The listing builds one solid part. Answer for the finished solid, in the listing's coordinates (mm). Face numbers are marked on the shaded views. A direction names the side the tool comes from. Give positions to 0.01 mm unless a question says otherwise; leave off trailing zeros. Order: outer loops, then holes, each group sorted by start corner. A loop starts at its lowest first (then second) coordinate and runs counter-clockwise, first axis right, second up. Notation, with made-up numbers: (69.5, 33) - (75.5, 33) arc R10 cw to (75.5, 39) - close; hole circle Ø9 at (48, 37). An arc over 180 degrees is marked (long way). Write each question's results on one line, items separated by ' | '. Start each with the question number.
1. Find the intervals of material crossed by L1, parallel to Y at x = 15, z = 3.5; L2, parallel to Y at x = 18.75, z = -3.25; L3, parallel to Y at x = 15, z = 2.5, in increasing order.
2. Section B-B (x = 15) is taken. Give the vertices of the cut face in (y, z).
3. Section A-A (y = 26) is taken. Give the vertices of the cut face in (x, z).
4. Flat-ended cylindrical pins translate along their axes: pin 1 (1.8 mm diameter, centred on x = 16, y = 21, fed in from -Z); pin 2 (3 mm diameter, centred on x = 15, y = 24, fed in from +Z); pin 3 (6.5 mm diameter, centred on y = -3.5, z = 1, fed in from -X); pin 4 (6 mm diameter, centred on y = 24, z = 4.5, fed in from +X). Find the tip coordinate at first contact, or state that the pin passes through.
5. Section D-D (x = 11.5) is taken. Give the vertices of the cut face in (y, z), and give its area (3 significant figures).
6. Determine the mould class of the marked faces 1, 2, 3 and 4 for opening direction Y: released by +Y, released by -Y, zero draft, split by the parting line, or undercut.
7. Which of the six approach directions +Z, -Z, +X, -X, +Y, -Y give full straight-line access (tool end or side, diameter ignored) to the marked faces 5, 6, 7, 8 and 9?
8. Section C-C (z = -0.5) is taken. Give the vertices of the cut face in (x, y).
Autodesk Inventor part; units mm, degrees
ref_plane "YZ Plane" through (0, 0, 0) normal (1, 0, 0) x (0, 1, 0)
ref_plane "XZ Plane" through (0, 0, 0) normal (0, 1, 0) x (-1, 0, 0)
ref_plane "XY Plane" through (0, 0, 0) normal (0, 0, 1) x (1, 0, 0)
sketch "스케치1" plane through (0, 0, 0) normal (0, 0, 1) x (1, 0, 0)
  line L0 (0, 0) -> (30, 0)
  line L1 (30, 0) -> (30, 20)
  line L2 (30, 20) -> (0, 20)
  line L3 (0, 20) -> (0, 0)
  line L4 (0, 20) -> (30, 20)
  line L5 (30, 20) -> (30, 17)
  line L6 (0, 17) -> (0, 20)
  line L7 (12, 20) -> (18, 20)
  line L8 (18, 20) -> (18, 16)
  line L9 (18, 16) -> (12, 16)
  line L10 (12, 16) -> (12, 20)
  point P0 (15, 20)
  point P1 (15, 20)
  dimension "d0" = 20
  dimension "d1" = 30
  dimension "d2" = 3
  dimension "d3" = 6
  dimension "d4" = 4
extrude "돌출1" add sketch "스케치1" along normal blind 10 contours L2 L8 L9 L10
sketch "스케치2" plane through (0, 0, 10) normal (0, 0, 1) x (1, 0, 0)
  line L0 (18, 20) -> (12, 20)
  line L1 (12, 20) -> (18, 20)
  line L2 (18, 20) -> (18, -3)
  line L3 (18, -3) -> (12, -3)
  line L4 (12, -3) -> (12, 20)
  point P0 (0, 0)
  dimension "d23" = 23
extrude "돌출2" add sketch "스케치2" along normal blind 4
sketch "스케치3" plane through (0, 0, 10) normal (0, 0, -1) x (-1, 0, 0)
  line L0 (-18, -3) -> (-18, 16)
  line L1 (-12, 16) -> (-12, -3)
  line L2 (-18, -3) -> (-12, -3)
  line L3 (-12, -3) -> (-12, 1)
  line L4 (-12, 1) -> (-18, 1)
  line L5 (-18, 1) -> (-18, -3)
  point P0 (0, 0)
  dimension "d9" = 4
extrude "돌출3" add sketch "스케치3" along normal blind 15
sketch "스케치6" plane through (0, 0, 0) normal (0, 0, -1) x (-1, 0, 0)
  line L0 (-18, 16) -> (-18, 20)
  line L1 (-12, 16) -> (-18, 16)
  line L2 (-12, 20) -> (-12, 16)
  line L3 (-18, 20) -> (-12, 20)
  line L4 (-18, 16) -> (-18, 20)
  line L5 (-18, 16) -> (-12, 16)
  line L6 (-12, 16) -> (-12, 36)
  line L7 (-12, 36) -> (-18, 36)
  line L8 (-18, 36) -> (-18, 16)
  point P0 (0, 0)
  dimension "d20" = 20
extrude "돌출6" add sketch "스케치6" against normal blind 4 contours L8 L7 L6 L3
sketch "스케치7" plane through (12, 1, 10) normal (0, 1, 0) x (1, 0, 0)
  line L0 (6, 0) -> (0, 0)
  line L1 (6, 0) -> (6, 15)
  line L2 (0, 15) -> (6, 15)
  line L3 (0, 0) -> (0, 15)
  line L4 (-4.5, 15) -> (10.5, 15)
  line L5 (10.5, 15) -> (10.5, 10)
  line L6 (10.5, 10) -> (-4.5, 10)
  line L7 (-4.5, 10) -> (-4.5, 15)
  point P0 (-12, 10)
  point P1 (3, 15)
  point P2 (3, 15)
  point P3 (6, 15)
  point P4 (6, 10)
  point P5 (0, 10)
  dimension "d27" = 15
extrude "돌출7" add sketch "스케치7" against normal blind 4 contours L1 L4 L5 L6 | L6 L7 L4 L3
sketch "스케치8" plane through (0, 0, -5) normal (0, 0, -1) x (-1, 0, 0)
  line L0 (-22.5, 1) -> (-7.5, 1)
  line L1 (-22.5, 1) -> (-22.5, -3)
  line L2 (-7.5, -3) -> (-22.5, -3)
  line L3 (-7.5, 1) -> (-7.5, -3)
  line L4 (-22.5, 1) -> (-7.5, 1)
  line L5 (-7.5, 1) -> (-7.5, -6)
  line L6 (-7.5, -6) -> (-22.5, -6)
  line L7 (-22.5, -6) -> (-22.5, 1)
  point P0 (0, 0)
  dimension "d28" = 7
extrude "돌출8" add sketch "스케치8" against normal blind 10
sketch "스케치9" plane through (0, 0, -5) normal (0, 0, -1) x (-1, 0, 0)
  line L0 (-20.1, 0.5) -> (-9.9, 0.5)
  line L1 (-9.9, 0.5) -> (-9.9, -4.5)
  line L2 (-9.9, -4.5) -> (-20.1, -4.5)
  line L3 (-20.1, -4.5) -> (-20.1, 0.5)
  line L4 (-22.5, 1) -> (-7.5, 1)
  line L5 (-22.5, 1) -> (-22.5, -6)
  point P0 (0, 0)
  point P1 (-15, 1)
  point P2 (-15, 0.5)
  dimension "d31" = 10.2
  dimension "d32" = 5
  dimension "d33" = 0.5
extrude "돌출9" cut sketch "스케치9" against normal blind 8
sketch "스케치10" plane through (0, 0, -5) normal (0, 0, -1) x (-1, 0, 0)
  line L0 (-9.9, 0.5) -> (-9.9, -4.5)
  line L1 (-9.9, -4.5) -> (-20.1, -4.5)
  line L2 (-20.1, -4.5) -> (-20.1, 0.5)
  line L3 (-20.1, 0.5) -> (-9.9, 0.5)
  line L4 (-22.5, 1) -> (-7.5, 1)
  line L5 (-22.5, 1) -> (-22.5, -6)
  line L6 (-22.5, -6) -> (-7.5, -6)
  line L7 (-7.5, 1) -> (-7.5, -6)
  point P0 (0, 0)
extrude "돌출10" add sketch "스케치10" along normal blind 2
sketch "스케치11" plane through (12, 1, 10) normal (0, 1, 0) x (1, 0, 0)
  line L0 (0, 0) -> (0, 5)
  line L1 (6, 0) -> (0, 0)
  line L2 (6, 0) -> (6, 5)
  line L3 (10.5, 5) -> (6, 5)
  line L4 (10.5, 5) -> (10.5, 17)
  line L5 (-4.5, 17) -> (10.5, 17)
  line L6 (-4.5, 17) -> (-4.5, 5)
  line L7 (0, 5) -> (-4.5, 5)
  line L8 (-9.5, 11) -> (15.5, 11)
  line L9 (15.5, 11) -> (15.5, 17)
  line L10 (15.5, 17) -> (-9.5, 17)
  line L11 (-9.5, 17) -> (-9.5, 11)
  line L12 (0, 5) -> (6, 5)
  point P0 (-12, 10)
  point P1 (3, 11)
  point P2 (3, 5)
  point P3 (10.5, 17)
  point P4 (10.5, 11)
  point P5 (-4.5, 11)
  dimension "d39" = 25
  dimension "d40" = 6
extrude "돌출11" add sketch "스케치11" against normal blind 7 contours L8 L11 L10 L6 | L4 L10 L9 L8
sketch "스케치12" plane through (0, 0, 0) normal (0, 0, -1) x (-1, 0, 0)
  line L0 (-12, 16) -> (-12, 36)
  line L1 (-18, 16) -> (-18, 36)
  line L2 (-12, 16) -> (-18, 16)
  line L3 (-12, 16) -> (-12, 36)
  line L4 (-12, 36) -> (-18, 36)
  point P0 (0, 0)
extrude "돌출12" cut sketch "스케치12" against normal blind 2
sketch "스케치13" plane through (0, 0, 4) normal (0, 0, 1) x (1, 0, 0)
  line L0 (18, 20) -> (18, 36)
  line L1 (18, 36) -> (12, 36)
  line L2 (12, 36) -> (12, 20)
  line L3 (18, 20) -> (12, 20)
  circle A0 centre (15, 33) radius 1.2
  circle A1 centre (15, 26) radius 1.2
  point P0 (0, 0)
  point P1 (15, 36)
  dimension "d45" = 2.4
  dimension "d48" = 3
  dimension "d51" = 7
extrude "돌출13" cut sketch "스케치13" against normal blind 2 contours A0 | A1
sketch "스케치16" plane through (0, 0, 2) normal (0, 0, -1) x (-1, 0, 0)
  circle A0 centre (-15, 19) radius 2.3
  line L0 (-12, 16) -> (-18, 16)
  point P0 (0, 0)
  point P1 (-15, 16)
  dimension "d59" = 4.6
  dimension "d60" = 3
properties part number "final522"
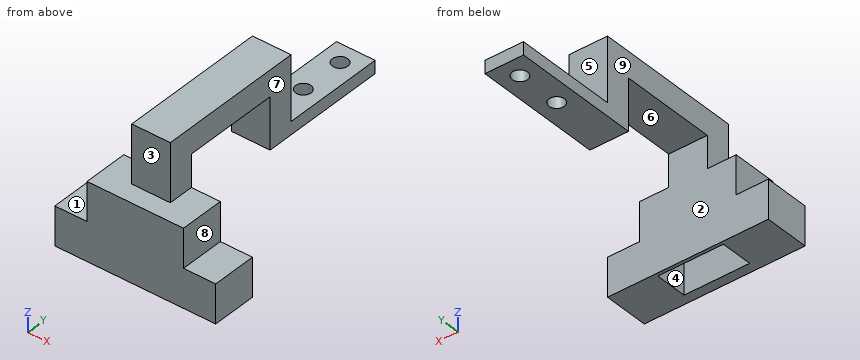
Reported:
1) L1: -6 to 1, 16 to 24.8, 27.2 to 31.8, 34.2 to 36 | L2: -6 to -4.5, 0.5 to 1 | L3: -6 to -4.5, 0.5 to 1, 16 to 24.8, 27.2 to 31.8, 34.2 to 36
2) outline: (-6, -7) - (-4.5, -7) - (-4.5, 3) - (0.5, 3) - (0.5, -7) - (1, -7) - (1, 10) - (16, 10) - (16, 2) - (24.8, 2) - (24.8, 4) - (20, 4) - (20, 14) - (-3, 14) - (-3, 5) - (-6, 5) - close; (27.2, 2) - (31.8, 2) - (31.8, 4) - (27.2, 4) - close; (34.2, 2) - (36, 2) - (36, 4) - (34.2, 4) - close
3) outline: (12, 2) - (13.8, 2) - (13.8, 4) - (12, 4) - close; (16.2, 2) - (18, 2) - (18, 4) - (16.2, 4) - close
4) pin 1: z = 2 | pin 2: z = 4 | pin 3: x = 2.5 | pin 4: x = 18
5) outline: (-6, -7) - (-4.5, -7) - (-4.5, 3) - (0.5, 3) - (0.5, -7) - (1, -7) - (1, 5) - (-6, 5) - close | area: 34.0 mm²
6) face 1: zero draft | face 2: undercut | face 3: released by -Y | face 4: undercut
7) face 5: +Z, +X, -X, +Y | face 6: -Z, +X, -X | face 7: +Z, +X, +Y | face 8: +Z, +X, +Y, -Y | face 9: +Z, -X, +Y
8) outline: (7.5, -6) - (22.5, -6) - (22.5, 1) - (7.5, 1) - close; hole (9.9, -4.5) - (20.1, -4.5) - (20.1, 0.5) - (9.9, 0.5) - close
